Can you work these out from the drawing? Everything is in mm from the part's minimum corner. Round coordinates to 2 decimals unless told otherwise and drop trailing zeros. Loops run counter-clockwise (first coordinate to the right, second up) from the corner with the lowest first, then second, coordinate; pieces in that order, holes last. Notation, with made-up numbers: (-39, 35) -> (-5, 35) arc R12 cw to (-5, 53) -> close; hole circle Ø11 at (-8, 65.25). An arc over 180 degrees is marked (long way). One line per item, written item: value.
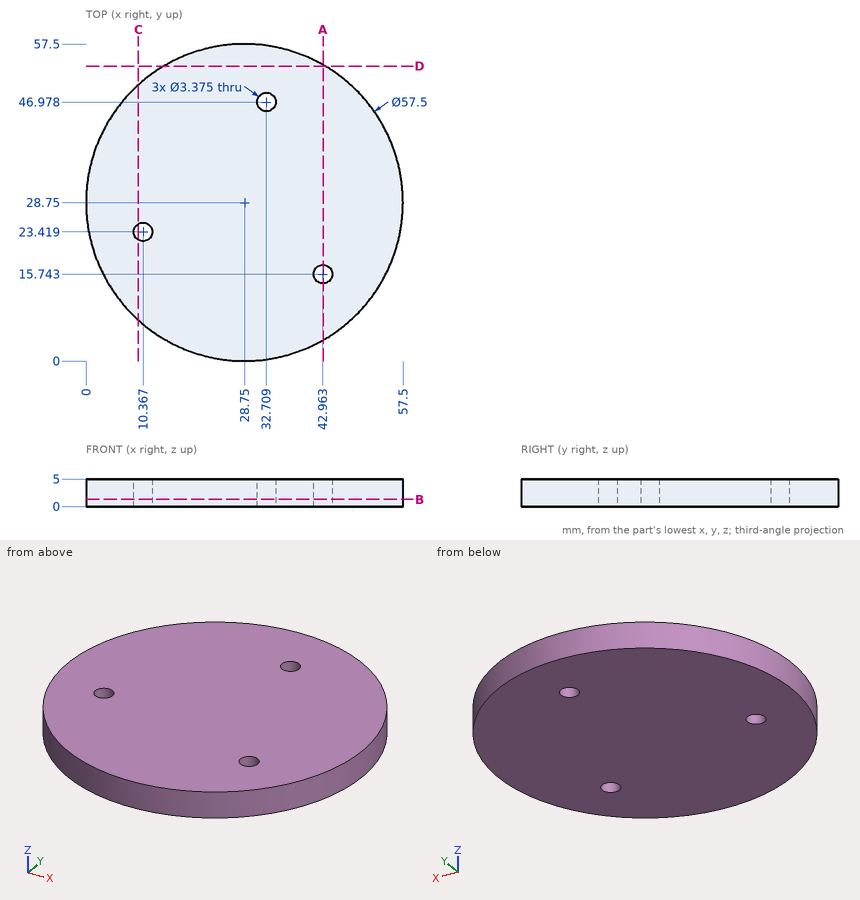
(1) If we section it at C-C, the plane x = 9.5: Please give me the cut outline in (y, z) (1 decimal), then the cut area to 3 significant figures.
Recorded:
outline: (7.4, 0) -> (22, 0) -> (22, 5) -> (7.4, 5) -> close; (24.9, 0) -> (50.1, 0) -> (50.1, 5) -> (24.9, 5) -> close
area: 199 mm²
(2) If we section it at D-D, the plane y = 53.5: Please give me the cut outline in (x, z), then the cut area to 3 significant figures.
Recorded:
outline: (14.12, 0) -> (43.38, 0) -> (43.38, 5) -> (14.12, 5) -> close
area: 146 mm²
(3) If I drill on L1, parallel to X at y = 24.5, z = 2.6 (1 decimal); L2, parallel to Y at x = 11, z = 0.4 (1 decimal); L3, parallel to Y at x = 9, z = 4.05 (1 decimal), over which ranges is the centre line in solid material (lowest first)?
Recorded:
L1: 0.3 to 9.1, 11.7 to 57.2
L2: 6.1 to 21.9, 25 to 51.4
L3: 7.9 to 22.4, 24.4 to 49.6
(4) If we section it at A-A, the plane x = 43: Please give me the cut outline in (y, z) (1 decimal), then the cut area to 3 significant figures.
Recorded:
outline: (3.8, 0) -> (14.1, 0) -> (14.1, 5) -> (3.8, 5) -> close; (17.4, 0) -> (53.7, 0) -> (53.7, 5) -> (17.4, 5) -> close
area: 233 mm²
(5) If we section it at B-B, the plane z = 1.3: Give the number of separate pieces and of enclosed holes in the cut face, then the cut area to 3 significant figures.
Recorded:
separate pieces: 1
enclosed holes: 3
area: 2,570 mm²
(6) I'm going to push flat-ended pins straight in: pin 1 Ø1.5 at (y, z) = (24, 4.5) entering from -X; pin 2 Ø3 at (y, z) = (36, 4.5) entering from -X; pin 3 Ø1.5 at (x, z) = (50.5, 3.5) entering from -Y (1 decimal). Where does each tip first touch, or does it pass through?
Recorded:
pin 1: x = 0.28
pin 2: x = 0.58
pin 3: y = 9.1
